For this review, take the finished solid that the model builds, in its own axes (mm). Coordinates: 2 decimals unless noted, no trailing zeros. Write each loop counter-clockwise with the first axis right and the second up, starting at its lowest first coordinate (ties: lowest second). Pieces come first, ordered by that corner, then holes.
```python
from build123d import *

# Parameters (mm, degrees)
F0_W     = 25.4
F0_H     = 25.4
F1_DEPTH = 736.6
F2_W     = 22.2504
F2_H     = 22.2504
F3_DEPTH = 736.6
F4_R     = 1.524
F5_R     = 0.254


with BuildPart() as f1:
    # F0 (on Front) → F1 (new body)
    with BuildSketch(Plane.XZ):
        Rectangle(F0_W, F0_H)
    extrude(amount=F1_DEPTH)

    # F2 (on face) → F3 (cut, through all)
    with BuildSketch(Plane.XZ.offset(736.6)):
        Rectangle(F2_W, F2_H)
    extrude(amount=-F3_DEPTH, mode=Mode.SUBTRACT)

    # F4
    f4_edges = [f1.edges().sort_by_distance(p)[0] for p in [
        (-11.1252, -368.3, 11.1252),
        (11.1252, -368.3, -11.1252),
        (11.1252, -368.3, 11.1252),
        (-11.1252, -368.3, -11.1252),
    ]]
    fillet(f4_edges, radius=F4_R)

    # F5
    f5_edges = [f1.edges().sort_by_distance(p)[0] for p in [
        (12.7, -368.3, 12.7),
        (12.7, -368.3, -12.7),
        (-12.7, -368.3, -12.7),
        (-12.7, -368.3, 12.7),
    ]]
    fillet(f5_edges, radius=F5_R)


solid = f1.part
```
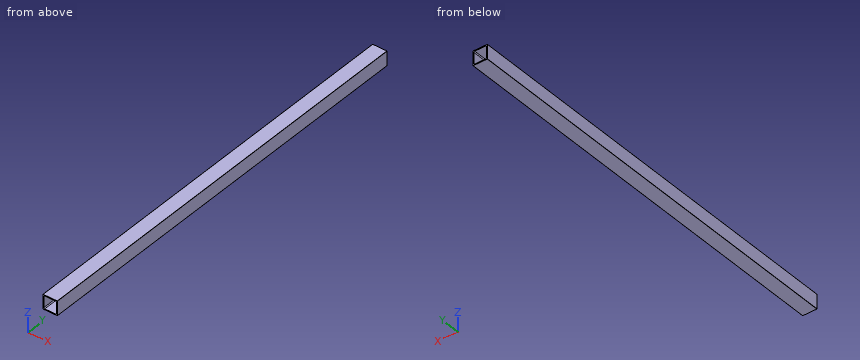
Q1. For probe 1 along X at (y, z) = (-240.5, 7.75); probe 2 along Z at (x, y) = (-10, -599.5); probe 3 along X at (y, z) = (-266, -10.5), list the stretches that pass through material, from the lowest coordinate up.
Ans:
probe 1: x = -12.7 to -11.13, 11.13 to 12.7
probe 2: z = -12.7 to -11.07, 11.07 to 12.7
probe 3: x = -12.7 to -10.83, 10.83 to 12.7
Q2. Clearance check with a flat-ended pin moving along its axis: pin 1 Ø1.5 at (x, z) = (8.5, -7.5) entering from -Y. State where the tip first meets the part, or that it passes through.
Ans:
pin 1: passes through
Q3. Add section C-C (y = -332.5). State the section outline as (x, z) points.
Ans:
outline: (-12.7, -12.45) arc R0.25 ccw to (-12.45, -12.7) - (12.45, -12.7) arc R0.25 ccw to (12.7, -12.45) - (12.7, 12.45) arc R0.25 ccw to (12.45, 12.7) - (-12.45, 12.7) arc R0.25 ccw to (-12.7, 12.45) - close; hole (-11.13, -9.6) arc R1.52 ccw to (-9.6, -11.13) - (9.6, -11.13) arc R1.52 ccw to (11.13, -9.6) - (11.13, 9.6) arc R1.52 ccw to (9.6, 11.13) - (-9.6, 11.13) arc R1.52 ccw to (-11.13, 9.6) - close
Q4. Add section B-B (x = -4.5). State the section outline as (y, z) points.
Ans:
outline: (-736.6, -12.7) - (0, -12.7) - (0, -11.13) - (-736.6, -11.13) - close; (-736.6, 11.13) - (0, 11.13) - (0, 12.7) - (-736.6, 12.7) - close
Q5. Add section A-A (z = -3.75). State the section outline as (x, y) points, then the cut area to 3 significant figures.
Ans:
outline: (-12.7, -736.6) - (-11.13, -736.6) - (-11.13, 0) - (-12.7, 0) - close; (11.13, -736.6) - (12.7, -736.6) - (12.7, 0) - (11.13, 0) - close
area: 2,320 mm2
